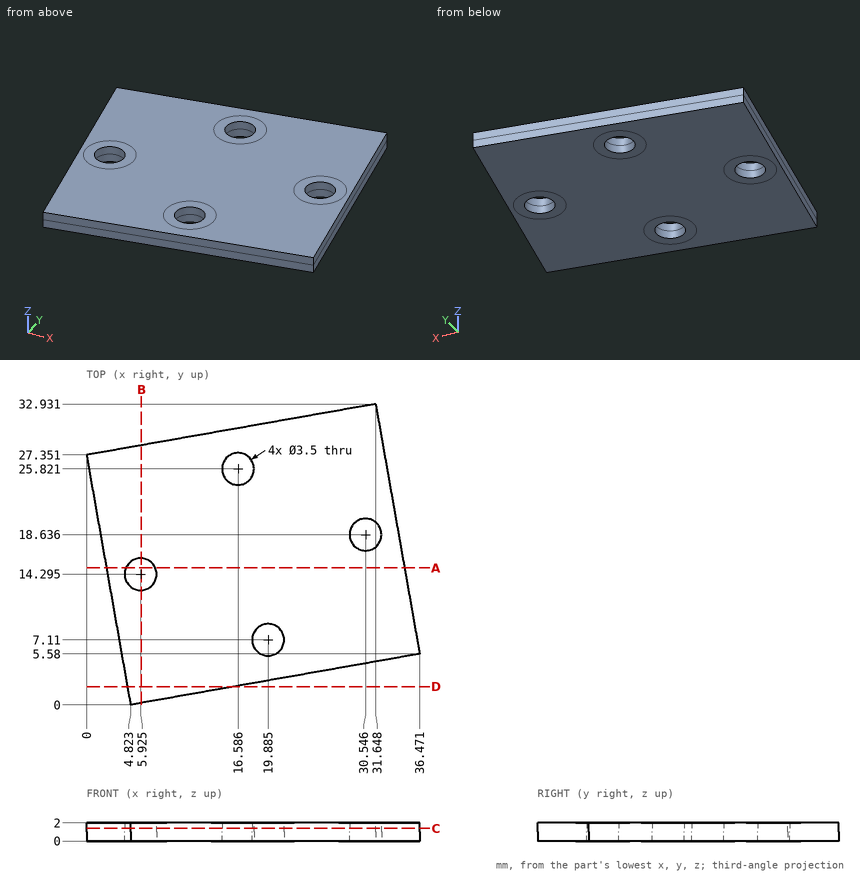
Geometry: see drawing. Coordinates: mm, zero at the bounding-box minimum. Give positions to 0.01 mm unless a question says otherwise; leave off trailing zeros. Write each loop counter-clockwise with the first axis right and the second up, starting at its lowest first coordinate (ties: lowest second). Pieces come first, ordered by that corner, then holes. Notation, with made-up numbers: M 16.5,-39 L 64.5,-39 A23 ccw 64.5,-15 Z; hole C 40.5,67 d4. An arc over 180 degrees is marked long. Answer in a Markdown table with one row per item. Add a question column.
(1) Ray query, line 1 (Y direction, x = 20, z = 1.4) (1 decimal); line 2 (Y direction, x = 16.5, z = 0.35); line 3 (X direction, y = 8, z = 1.9) (1 decimal). Return the intervals inside material, ascending.
(2) Section D-D on y = 2. Return loops of the section in (x, z) (1 decimal).
(3) Section B-B on x = 6. Return loops of the section in (y, z).
(4) Section A-A on y = 15. Return loops of the section in (x, z).
(5) First-contact query: pin 1 (1 mm diameter, centred on y = 7, z = 1, fed in from +X). Flat tip, straight axial feed; report the tip coordinate or a pass-through.
(6) Section C-C on z = 1.4. State how many separate pieces and enclosed holes the cut face has, and give its area (3 significant figures).
Result set:
| question | item | result |
|---|---|---|
| 1 | line 1 | y = 2.7 to 5.4, 8.9 to 30.9 |
| 1 | line 2 | y = 2.06 to 24.07, 27.57 to 30.26 |
| 1 | line 3 | x = 3.4 to 18.4, 21.4 to 36 |
| 2 | outline | M 4.5,0 L 16.2,0 L 16.2,2 L 4.5,2 Z |
| 3 | outline | M 0.21,0 L 12.55,0 L 12.55,2 L 0.21,2 Z; M 16.04,0 L 28.41,0 L 28.41,2 L 16.04,2 Z |
| 4 | outline | M 2.18,0 L 4.32,0 L 4.32,2 L 2.18,2 Z; M 7.53,0 L 34.81,0 L 34.81,2 L 7.53,2 Z |
| 5 | pin 1 | stops at x = 36.31 |
| 6 | separate pieces | 1 |
| 6 | enclosed holes | 4 |
| 6 | area | 854 mm^2 |
